```python
from build123d import *

# Parameters (mm, degrees)
DODANIE_WYCI_GNI_CIE1_START = 27.457167
DODANIE_WYCI_GNI_CIE1_DEPTH = 43.457167
SZKIC2_OUTSIDE_W            = 57.065
SZKIC2_OUTSIDE_H            = 51.608
WYTNIJ_WYCI_GNI_CIE1_DEPTH  = 35.037273975
SZKIC2_4_R                  = 12.5
SZKIC2_4_R_2                = 9
WYTNIJ_WYCI_GNI_CIE2_DEPTH  = 3
SZKIC2_5_R                  = 9
WYTNIJ_WYCI_GNI_CIE3_DEPTH  = 35.037274287
SFAZOWANIE1_SIZE            = 2
DODANIE_WYCI_GNI_CIE2_START = 22
DODANIE_WYCI_GNI_CIE2_DEPTH = 22
ZAOKR_GLENIE1_START         = -22
ZAOKR_GLENIE1_DEPTH         = 22
WYTNIJ_WYCI_GNI_CIE4_DEPTH  = 45.484784375
SZKIC8_R                    = 3.5
DODANIE_WYCI_GNI_CIE3_DEPTH = 1


with BuildPart() as part:
    # Szkic1 → Dodanie-wyciągnięcie1 (new body)
    with BuildSketch(Plane.XY.offset(DODANIE_WYCI_GNI_CIE1_START)):
        Polygon((4, 13.2), (2, 13.2), (2, 19.2), (0, 19.2), (0, -18.8), (2, -18.8), (2, -15.8), (4, -15.8), (4, -18), (6, -18), (6, 19.2), (4, 19.2), align=None)
    extrude(amount=-DODANIE_WYCI_GNI_CIE1_DEPTH)

    # Szkic2 outside → Wytnij-wyciągnięcie1 (cut, through all)
    with BuildSketch(Plane(origin=(0, 0, 0), x_dir=(0, 0, -1), z_dir=(1, 0, 0))):
        with Locations((-5.7285, 0.2)):
            Rectangle(SZKIC2_OUTSIDE_W, SZKIC2_OUTSIDE_H)
        with BuildLine():
            Line((-22, -18.8), (-22, -3.514226))
            ThreePointArc((-22, -3.514226), (-23.38343065, 8.166064436), (-27.457167387, 19.2))
            Line((-27.457167387, 19.2), (8.506468127, 19.2))
            ThreePointArc((8.506468127, 19.2), (12.568915153, 16.823268763), (16, 13.601470509))
            Line((16, 13.601470509), (16, -13.601470509))
            ThreePointArc((16, -13.601470509), (12.942371407, -16.537684915), (9.357350052, -18.8))
            Line((9.357350052, -18.8), (-22, -18.8))
        make_face(mode=Mode.SUBTRACT)
    extrude(amount=WYTNIJ_WYCI_GNI_CIE1_DEPTH, mode=Mode.SUBTRACT)

    # Szkic2<4> → Wytnij-wyciągnięcie2 (cut)
    with BuildSketch(Plane(origin=(0, 0, 0), x_dir=(0, 0, -1), z_dir=(1, 0, 0))):
        Circle(SZKIC2_4_R)
        Circle(SZKIC2_4_R_2, mode=Mode.SUBTRACT)
    extrude(amount=WYTNIJ_WYCI_GNI_CIE2_DEPTH, mode=Mode.SUBTRACT)

    # Szkic2<5> → Wytnij-wyciągnięcie3 (cut, through all)
    with BuildSketch(Plane(origin=(0, 0, 0), x_dir=(0, 0, -1), z_dir=(1, 0, 0))):
        with Locations(Location((0, 0, 0), (0, 0, 180))):
            Circle(SZKIC2_5_R)
    extrude(amount=WYTNIJ_WYCI_GNI_CIE3_DEPTH, mode=Mode.SUBTRACT)

    # Sfazowanie1
    # the kernel refuses this chamfer: 2 mm, written as the material it takes off along each edge
    with BuildSketch(Plane(origin=(4, 13.2, -16), x_dir=(0, 0, 1), z_dir=(-1, 0, 0))) as sfazowanie1_piece_1:
        Polygon((SFAZOWANIE1_SIZE, 0), (0, -SFAZOWANIE1_SIZE), (0, 0), align=None)
    extrude(amount=2, mode=Mode.SUBTRACT)
    with BuildSketch(Plane(origin=(4, -15.8, -13.833293173), x_dir=(0, 0, 1), z_dir=(-1, 0, 0))) as sfazowanie1_piece_2:
        with BuildLine():
            Line((0.773430999, 0), (-0.601291335, 0.547368421))
            ThreePointArc((-0.601291335, 0.547368421), (-0.33094721, 0.295991022), (0, 0))
            Line((0, 0), (0.773430999, 0))
        make_face()
    extrude(amount=2, mode=Mode.SUBTRACT)

    # Szkic3 → Dodanie-wyciągnięcie2 (add)
    with BuildSketch(Plane.ZY.offset(DODANIE_WYCI_GNI_CIE2_START)):
        with BuildLine():
            Line((-18, -10.816653826), (-18, 0))
            ThreePointArc((-18, 0), (0, -18), (18, 0))
            Line((18, 0), (18, -10.816653826))
            ThreePointArc((18, -10.816653826), (0, -21), (-18, -10.816653826))
        make_face()
    extrude(amount=-DODANIE_WYCI_GNI_CIE2_DEPTH)

    # Zaokrąglenie1: read off the stored shape, not the designer's step
    # Zaokrąglenie1 outline → Zaokrąglenie1 (cut)
    with BuildSketch(Plane.YZ.offset(ZAOKR_GLENIE1_START)):
        with BuildLine():
            Line((-10.816653826, -18), (-9.327379053, -18))
            ThreePointArc((-9.327379053, -18), (-10.858310142, -17.759858191), (-12.242185007, -17.0625))
            ThreePointArc((-12.242185007, -17.0625), (-11.538944434, -17.545733423), (-10.816653826, -18))
        make_face()
        with BuildLine():
            ThreePointArc((-8.038687618, -16.105263158), (-7.511952847, -17.229415734), (-8.485281374, -18))
            Line((-8.485281374, -18), (0, -18))
            ThreePointArc((0, -18), (-4.12948321, -17.519913482), (-8.038687618, -16.105263158))
        make_face()
        with BuildLine():
            ThreePointArc((-10.816653826, 18), (-11.538944434, 17.545733423), (-12.242185007, 17.0625))
            ThreePointArc((-12.242185007, 17.0625), (-10.858310142, 17.759858191), (-9.327379053, 18))
            Line((-9.327379053, 18), (-10.816653826, 18))
        make_face()
        with BuildLine():
            ThreePointArc((-8.485281374, 18), (-7.511952847, 17.229415734), (-8.038687618, 16.105263158))
            ThreePointArc((-8.038687618, 16.105263158), (-4.12948321, 17.519913482), (0, 18))
            Line((0, 18), (-8.485281374, 18))
        make_face()
    extrude(amount=ZAOKR_GLENIE1_DEPTH, mode=Mode.SUBTRACT)

    # ZaawansowanyOtwór1: read off the stored shape, not the designer's step
    # ZaawansowanyOtwór1 outline → ZaawansowanyOtwór1 (revolve, cut)
    with BuildSketch(Plane(origin=(0, -10.606601718, 10.606601718), x_dir=(0, 1, 0), z_dir=(0, 0, -1))):
        Polygon((1.7, 3.84), (3.36, 5.5), (3.36, 6), (0, 6), (0, 0), (1.55, 0), (1.55, 3.84), align=None)
    revolve(axis=Axis((0, -10.606601718, 10.606601718), (1, 0, 0)), mode=Mode.SUBTRACT)

    # ZaawansowanyOtw_r1 2 outline → ZaawansowanyOtw_r1 2 (revolve, cut)
    with BuildSketch(Plane(origin=(0, -10.606601718, -10.606601718), x_dir=(0, 1, 0), z_dir=(0, 0, -1))):
        Polygon((3.36, 6), (0, 6), (0, 0), (1.55, 0), (1.55, 3.84), (1.7, 3.84), (3.36, 5.5), align=None)
    revolve(axis=Axis((0, -10.606601718, -10.606601718), (1, 0, 0)), mode=Mode.SUBTRACT)

    # ZaawansowanyOtw_r1 3 outline → ZaawansowanyOtw_r1 3 (revolve, cut)
    with BuildSketch(Plane(origin=(0, 10.606601718, -10.606601718), x_dir=(0, 1, 0), z_dir=(0, 0, -1))):
        Polygon((3.36, 6), (0, 6), (0, 0), (1.55, 0), (1.55, 3.84), (1.7, 3.84), (3.36, 5.5), align=None)
    revolve(axis=Axis((0, 10.606601718, -10.606601718), (1, 0, 0)), mode=Mode.SUBTRACT)

    # ZaawansowanyOtw_r1 4 outline → ZaawansowanyOtw_r1 4 (revolve, cut)
    with BuildSketch(Plane(origin=(0, 10.606601718, 10.606601718), x_dir=(0, 1, 0), z_dir=(0, 0, -1))):
        Polygon((3.36, 6), (0, 6), (0, 0), (1.55, 0), (1.55, 3.84), (1.7, 3.84), (3.36, 5.5), align=None)
    revolve(axis=Axis((0, 10.606601718, 10.606601718), (1, 0, 0)), mode=Mode.SUBTRACT)

    # Szkic7 → Wytnij-wyciągnięcie4 (cut, through all)
    with BuildSketch(Plane(origin=(6, 0, 0), x_dir=(0, 0, -1), z_dir=(1, 0, 0))):
        with BuildLine():
            Line((-23, 17.75), (-13, 17.75))
            ThreePointArc((-13, 17.75), (-11.45, 16.2), (-13, 14.65))
            Line((-13, 14.65), (-23, 14.65))
            ThreePointArc((-23, 14.65), (-24.55, 16.2), (-23, 17.75))
        make_face()
    extrude(amount=-WYTNIJ_WYCI_GNI_CIE4_DEPTH, mode=Mode.SUBTRACT)

    # Szkic8 → Dodanie-wyciągnięcie3 (add)
    with BuildSketch(Plane.ZY):
        with Locations(Location((13, 16.2, 0), (0, 0, 58.997280866))):
            Circle(SZKIC8_R)
    extrude(amount=DODANIE_WYCI_GNI_CIE3_DEPTH)


solid = part.part
```
Source: CAD feature listing. Evaluate the final solid. Frame: model axes, mm. A direction names the side the tool comes from. Coordinates: 2 decimals unless noted, no trailing zeros. Write each loop counter-clockwise with the first axis right and the second up, starting at its lowest first coordinate (ties: lowest second). Pieces come first, ordered by that corner, then holes. Notation, with made-up numbers: M 48,78.25 L 58,78.25 A31 cw 58,112.25 Z; hole C 52.25,-20.5 d9. An arc over 180 degrees is marked long. Answer as a JSON object with one key per item and string values.
1. Contact query for flat-ended pins moving along their axis: P1, Ø2.5, axis at y = 11, z = -10, coming from the +X side; P2, Ø1.6, axis at x = 1, z = 11, coming from the +Y side; P3, Ø11, axis at y = -10.61, z = -10.61, coming from the -X side; P4, Ø4, axis at y = 10.61, z = 10.61, coming from the -X side. Output: stop coordinate, or through.
Evaluation:
{"P1": "x = 4.11", "P2": "y = 19.2", "P3": "x = -22", "P4": "x = 0"}
2. Ray query, L1, parallel to X at y = -16, z = -8; L2, parallel to Y at x = 3.9, z = 0; L3, parallel to Y at x = 1.35, z = 0. Return the intervals inside material, ascending.
Evaluation:
{"L1": "0 to 2, 4 to 6", "L2": "-15.8 to -9, 9 to 13.2", "L3": "-18.8 to -12.5, 12.5 to 19.2"}
3. Draft query along Y for faces 1 (the flat face through (3, -11, 22)), 2 (the flat face through (1, -18.8, 7)), 3 (the cylindrical face through (5.75, 13.71, -11.89)). Return one class per face: released by +Y, released by -Y, zero draft, split by the parting line, or undercut.
Evaluation:
{"face 1": "zero draft", "face 2": "released by -Y", "face 3": "undercut"}
4. Cut plane B-B on x = -3. Output: boundary loops of the cut face in (y, z), plus the area to 3 significant figures.
Evaluation:
{"outline": "M -12.24,-17.06 A5 ccw -9.33,-18 L -8.49,-18 A1 ccw -8.04,-16.11 A18 cw -8.04,16.11 A1 ccw -8.49,18 L -9.33,18 A5 ccw -12.24,17.06 A21 ccw Z", "area": "131 mm^2"}
5. Access query for faces 4 (the cylindrical face through (1.479, 3.755, -11.923)), 5 (the cylindrical face through (1.01, 16.17, 24.55)), 6 (the flat face through (-22, -18.2, 0.1)), 7 (the cylindrical face through (5.754, -11.335, -13.887)). Directions: +Z, -Z, +X, -X, +Y, -Y. A direction counts if a zero-diameter tool reaches every point of the face in a straight line with its end or side. Return the directions, or none.
Evaluation:
{"face 4": "-X", "face 5": "+X, -X", "face 6": "+Z, -Z, -X, +Y, -Y", "face 7": "+X"}
6. Cut plane D-D on y = 16.2. Output: boundary loops of the cut face in (x, z).
Evaluation:
{"outline": "M -1,9.5 L 0,9.5 L 0,-13.36 L 2,-13.36 L 2,11.45 L 0,11.45 L 0,16.5 L -1,16.5 Z; M 0,24.55 L 2,24.55 L 2,26.05 L 0,26.05 Z; M 4,-13.36 L 6,-13.36 L 6,11.45 L 4,11.45 Z; M 4,24.55 L 6,24.55 L 6,26.05 L 4,26.05 Z"}
7. Cut plane A-A on z = 0. Output: boundary loops of the cut face in (x, y), plus the area to 3 significant figures.
Evaluation:
{"outline": "M -22,-21 L 0,-21 L 0,-18.8 L 2,-18.8 L 2,-15.8 L 4,-15.8 L 4,-18 L 6,-18 L 6,-9 L 3,-9 L 3,-12.5 L 0,-12.5 L 0,-18 L -22,-18 Z; M 0,12.5 L 3,12.5 L 3,9 L 6,9 L 6,19.2 L 4,19.2 L 4,13.2 L 2,13.2 L 2,19.2 L 0,19.2 Z", "area": "145 mm^2"}
8. Cut plane C-C on y = 1. Output: boundary loops of the cut face in (x, z), plus the area to 3 significant figures.
Evaluation:
{"outline": "M 0,-16 L 6,-16 L 6,-8.94 L 3,-8.94 L 3,-12.46 L 0,-12.46 Z; M 0,12.46 L 3,12.46 L 3,8.94 L 6,8.94 L 6,22.2 L 0,22.2 Z", "area": "101 mm^2"}
